Could you check a few things on this model? Use its own coordinates, in mm. Face numbers are marked on the shaded views. A direction names the side the tool comes from. Coordinates: 2 decimals unless noted, no trailing zeros. Order: outer loops, then holes, each group sorted by start corner. A loop starts at its lowest first (then second) coordinate and runs counter-clockwise, first axis right, second up. Notation, with made-up numbers: (-17, 26.25) - (20, 26.25) arc R28 ccw to (20, 62.25) - close; hole circle Ø4 at (57.5, 44). An arc over 180 degrees is marked (long way). One line per item, written item: value.
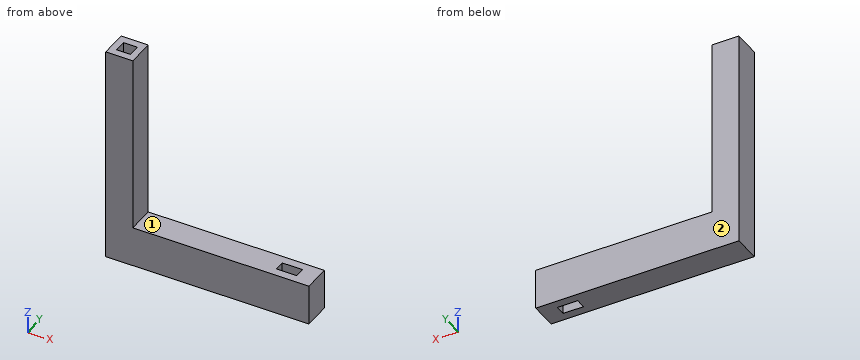
Autodesk Fusion 360 part; units mm, degrees
sketch "Esquisse1" plane through (0, 0, 0) normal (0, 0, 1) x (1, 0, 0)
  line L0 (0, 0) -> (8, 0)
  line L1 (8, 0) -> (8, 8)
  line L2 (8, 8) -> (0, 8)
  line L3 (0, 8) -> (0, 0)
  dimension "d1" = 8
  dimension "d2" = 8
extrude "Extrusion1" add sketch "Esquisse1" along normal blind 65
sketch "Esquisse8" plane through (0, 0, 65) normal (0, 0, 1) x (-1, 0, 0)
  line L0 (0, -8) -> (0, 0)
  line L1 (0, 0) -> (-8, 0)
  line L2 (-8, 0) -> (-8, -8)
  line L3 (-8, -8) -> (0, -8)
  line L4 (0, -4) -> (-8, -4)
  line L5 (-1.95, -4) -> (-6.05, -4)
  line L6 (-6.05, -4) -> (-6.05, -5.8)
  line L7 (-6.05, -5.8) -> (-1.95, -5.8)
  line L8 (-1.95, -5.8) -> (-1.95, -4)
  line L9 (-4, -8) -> (-4, 0)
  line L10 (-1.95, -2.2) -> (-1.95, -4)
  line L11 (-6.05, -2.2) -> (-1.95, -2.2)
  line L12 (-6.05, -4) -> (-6.05, -2.2)
  dimension "d41" = 4.1
  dimension "d42" = 2.05
  dimension "d43" = 1.8
extrude "Extrusion8" cut sketch "Esquisse8" against normal blind 6 contours L4 L5 L7 L8 L9 | L4 L5 L9 L10 L11 | L4 L5 L6 L7 L9 | L4 L5 L9 L11 L12
sketch "Esquisse9" plane through (8, 0, 0) normal (1, 0, 0) x (0, 1, 0)
  line L0 (0, 0) -> (8, 0)
  line L1 (8, 0) -> (8, 65)
  line L2 (8, 65) -> (0, 65)
  line L3 (0, 65) -> (0, 0)
  line L4 (0, 0) -> (8, 0)
  line L5 (8, 0) -> (8, 12)
  line L6 (8, 12) -> (0, 12)
  line L7 (0, 12) -> (0, 0)
  dimension "d46" = 12
extrude "Extrusion9" add sketch "Esquisse9" along normal blind 52 contours L0 L1 L3 L4 L5 L6 L7
sketch "Esquisse10" plane through (0, 0, 12) normal (0, 0, 1) x (-1, 0, 0)
  line L0 (-8, -8) -> (-8, 0)
  line L1 (-8, 0) -> (-60, 0)
  line L2 (-60, 0) -> (-60, -8)
  line L3 (-60, -8) -> (-8, -8)
  line L4 (-55, -5.5) -> (-49, -5.5)
  line L5 (-49, -5.5) -> (-49, -2.5)
  line L6 (-49, -2.5) -> (-55, -2.5)
  line L7 (-55, -2.5) -> (-55, -5.5)
  dimension "d49" = 2.5
  dimension "d50" = 2.5
  dimension "d51" = 5
  dimension "d52" = 6
extrude "Extrusion10" cut sketch "Esquisse10" against normal blind 23 contours L4 L5 L6 L7
Item 1: I want a section at C-C on y = 1.25. Please give me the cut outline in (x, z), then the cut area to 3 significant figures.
Conclusion:
outline: (0, 0) - (60, 0) - (60, 12) - (8, 12) - (8, 65) - (0, 65) - close
area: 1,140 mm²
Item 2: I want a section at B-B on y = 4.75. Please give me the cut outline in (x, z), then the cut area to 3 significant figures.
Conclusion:
outline: (0, 0) - (49, 0) - (49, 12) - (8, 12) - (8, 65) - (6.05, 65) - (6.05, 59) - (1.95, 59) - (1.95, 65) - (0, 65) - close; (55, 0) - (60, 0) - (60, 12) - (55, 12) - close
area: 1,050 mm²
Item 3: For the marked faces 1 and 2, which set-ups out of +Z, -Z, +X, -X, +Y, -Y let a thin tool reach every point of the face, with its end or its side?
Conclusion:
face 1: +Z, +X, +Y, -Y
face 2: +Z, -Z, +X, -X, +Y
Item 4: If I drill on probe 1 along X at (y, z) = (6.25, 52); probe 2 along Z at (x, y) = (35.5, 1.75); probe 3 along X at (y, z) = (4.25, 7), over which ranges is the centre line in solid material (lowest first)?
Conclusion:
probe 1: 0 to 8
probe 2: 0 to 12
probe 3: 0 to 49, 55 to 60
Item 5: I want a section at A-A on z = 8. Please give me the cut outline in (x, y), then the cut area to 3 significant figures.
Conclusion:
outline: (0, 0) - (60, 0) - (60, 8) - (0, 8) - close; hole (49, 2.5) - (55, 2.5) - (55, 5.5) - (49, 5.5) - close
area: 462 mm²
Item 6: I want a section at D-D on z = 45. Please give me the cut outline in (x, y).
Conclusion:
outline: (0, 0) - (8, 0) - (8, 8) - (0, 8) - close
Item 7: I'm going to push flat-ended pins straight in: pin 1 Ø1.8 at (x, y) = (4, 3.5) entering from +Z; pin 2 Ø1.1 at (y, z) = (3.5, 60.5) entering from -X; pin 3 Ø4 at (x, y) = (29, 3.5) entering from +Z; pin 4 Ø3 at (y, z) = (1.5, 58) entering from +X. Where does each tip first touch, or does it pass through?
Conclusion:
pin 1: z = 59
pin 2: x = 0
pin 3: z = 12
pin 4: x = 8
